Input: part model. Units: mm. Frame: model coordinates. Face numbers are marked on the shaded views. Round coordinates to 2 decimals unless told otherwise and drop trailing zeros. Write each loop counter-clockwise with the first axis right and the second up, starting at its lowest first coordinate (ties: lowest second). Pieces come first, ordered by that corner, then holes. Notation, with made-up numbers: (-10.5, 34) - (-0.5, 34) arc R27 cw to (-0.5, 72) - close; hole circle Ø10 at (1.5, -22.5). An arc over 180 degrees is marked (long way). Use one line per item in the form item = value.
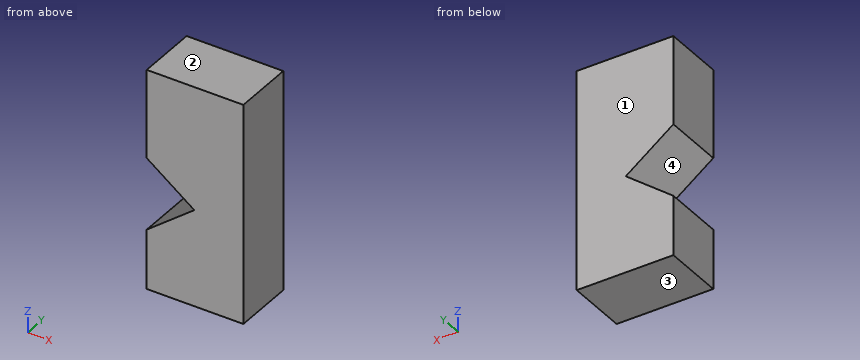
Autodesk Inventor part; units mm, degrees
ref_plane "YZ Plane" through (0, 0, 0) normal (1, 0, 0) x (0, 1, 0)
ref_plane "XZ Plane" through (0, 0, 0) normal (0, 1, 0) x (-1, 0, 0)
ref_plane "XY Plane" through (0, 0, 0) normal (0, 0, 1) x (1, 0, 0)
sketch "Sketch1" plane through (0, 0, 0) normal (0, 1, 0) x (-1, 0, 0)
  line L0 (-4.019, -7.9168) -> (3.8978, -7.9168)
  line L1 (3.8978, -7.9168) -> (3.8978, 10.1384)
  line L2 (3.8978, 10.1384) -> (-4.019, 10.1384)
  line L3 (-4.019, 10.1384) -> (-4.019, -7.9168)
  point P0 (0, 0)
extrude "Extrusion1" add sketch "Sketch1" along normal blind 5
sketch "Sketch2" plane through (0, 5, 0) normal (0, 1, 0) x (1, 0, 0)
  line L0 (-3.8978, -2.87) -> (0, 0)
  line L1 (0, 0) -> (-3.8978, 3.0252)
  line L2 (4.019, 7.9168) -> (-3.8978, 7.9168)
  line L3 (-3.8978, 7.9168) -> (-3.8978, -10.1384)
  line L4 (-3.8978, -10.1384) -> (4.019, -10.1384)
  line L5 (4.019, -10.1384) -> (4.019, 7.9168)
extrude "Extrusion2" cut sketch "Sketch2" against normal blind 5 contours L3 L1 L0
properties part number "Notch_example"
(1) Cut plane D-D on z = -0.25. Output: boundary loops of the cut face in (x, y), then the cut area to 3 significant figures.
Derived:
outline = (-0.32, 0) - (4.02, 0) - (4.02, 5) - (-0.32, 5) - close
area = 21.7 mm^2
(2) Draft query along Z for the marked faces 1, 2, 3 and 4. Return one class per face: released by +Z, released by -Z, zero draft, split by the parting line, or undercut.
Derived:
face_1 = zero draft
face_2 = released by +Z
face_3 = released by -Z
face_4 = undercut
(3) Cut plane C-C on x = -2.25. Output: boundary loops of the cut face in (y, z).
Derived:
outline = (0, -7.92) - (5, -7.92) - (5, -1.75) - (0, -1.75) - close; (0, 1.66) - (5, 1.66) - (5, 10.14) - (0, 10.14) - close
(4) Cut plane B-B on y = 2.35. Output: boundary loops of the cut face in (x, z), then the cut area to 3 significant figures.
Derived:
outline = (-3.9, -7.92) - (4.02, -7.92) - (4.02, 10.14) - (-3.9, 10.14) - (-3.9, 2.87) - (0, 0) - (-3.9, -3.03) - close
area = 131 mm^2
(5) Cut plane A-A on x = -3.5. Output: boundary loops of the cut face in (y, z).
Derived:
outline = (0, -7.92) - (5, -7.92) - (5, -2.72) - (0, -2.72) - close; (0, 2.58) - (5, 2.58) - (5, 10.14) - (0, 10.14) - close
(6) Material intervals for L1, parallel to Z at x = -2.5, y = 0.65; L2, parallel to Z at x = -2.75, y = 3.7; L3, parallel to X at y = 1.1, z = 0.25, sorted ascending.
Derived:
L1 = -7.92 to -1.94, 1.84 to 10.14
L2 = -7.92 to -2.13, 2.02 to 10.14
L3 = -0.34 to 4.02
